Autodesk Inventor part; units mm, degrees
ref_plane "YZ Plane" through (0, 0, 0) normal (1, 0, 0) x (0, 1, 0)
ref_plane "XZ Plane" through (0, 0, 0) normal (0, 1, 0) x (-1, 0, 0)
ref_plane "XY Plane" through (0, 0, 0) normal (0, 0, 1) x (1, 0, 0)
sketch "Sketch1" plane through (0, 0, 0) normal (0, 0, 1) x (1, 0, 0)
  circle A0 centre (0, 0) radius 6
  dimension "d0" = 12
extrude "Extrusion1" add sketch "Sketch1" along normal blind 50
sketch "Sketch2" plane through (0, 0, 50) normal (0, 0, 1) x (1, 0, 0)
  point P0 (0, 0)
chamfer "Chamfer1" distance 3 angle 45 1 edges at (-6, 0, 0)
sketch "Sketch4" plane through (0, 0, 0) normal (0, 0, -1) x (-1, 0, 0)
  circle A0 centre (0, 0) radius 2
  dimension "d8" = 4
extrude "Extrusion3" cut sketch "Sketch4" against normal blind 10
properties part number "arm"
Model file for the job. Use its own axes, mm. A direction names the side the tool comes from. Give positions to 0.01 mm unless a question says otherwise; leave off trailing zeros. Loops run counter-clockwise (first coordinate to the right, second up) from the corner with the lowest first, then second, coordinate; pieces in that order, holes last.
1) Saw through at A-A (y = 0). Write the cut outline in (x, z).
2) Pull direction Y, two halves, no side cores. Call faces 1 (the cylindrical face through (-6, 0, 26)), 2 (the flat face through (1, -2, 0)), 3 (the flat face through (0, 0, 10)): +Y half, -Y half, draft (parallel to the pull), parting line (faces both ways), or undercut.
3) Saw through at D-D (z = 23). Write the cut outline in (x, y), plus the area to 3 significant figures.
4) Saw through at B-B (z = 9.5). Write the cut outline in (x, y), plus the area to 3 significant figures.
5) Tool access for faces 4 (the flat face through (0, 0, 50)), 5 (the cylindrical face through (0, -2, 5)): list every direction of +Z, -Z, +X, -X, +Y, -Y with a clear straight run to the whole face (end or side of a thin tool).
6) Wall check: line 1 (Y direction, x = 0, z = 6); line 2 (Z direction, x = 0.5, y = 1.5); line 3 (Y direction, x = 0, z = 2.5). Give the ranges that are in metal, low to high.
7) Flat gauge pins, fed straight in: pin 1 Ø5 at (x, z) = (-4.5, 22.5) entering from -Y; pin 2 Ø2.5 at (x, y) = (0, 0) entering from -Z; pin 3 Ø2 at (x, z) = (1, 13.5) entering from -Y; pin 4 Ø6 at (y, z) = (4, 27) entering from +X. Where does each tip first touch, or does it go through?
Answer block:
1. outline: (-6, 3) - (-3, 0) - (-2, 0) - (-2, 10) - (2, 10) - (2, 0) - (3, 0) - (6, 3) - (6, 50) - (-6, 50) - close
2. face 1: parting line
2. face 2: draft
2. face 3: undercut
3. outline: circle Ø12 at (0, 0)
3. area: 113 mm2
4. outline: circle Ø12 at (0, 0); hole circle Ø4 at (0, 0)
4. area: 101 mm2
5. face 4: +Z, +X, -X, +Y, -Y
5. face 5: -Z
6. line 1: y = -6 to -2, 2 to 6
6. line 2: z = 10 to 50
6. line 3: y = -5.5 to -2, 2 to 5.5
7. pin 1: stops at y = -5.66
7. pin 2: stops at z = 10
7. pin 3: stops at y = -6
7. pin 4: stops at x = 5.92
